Read the model definition and answer for the solid it produces. Units are mm, in the model's axes. Face numbers are marked on the shaded views. Give positions to 0.01 mm unless a question says otherwise; leave off trailing zeros. Order: outer loops, then holes, each group sorted by start corner. A loop starts at its lowest first (then second) coordinate and runs counter-clockwise, first axis right, second up. Notation, with made-up numbers: (-34.75, 55.25) - (-16.75, 55.25) arc R11 cw to (-16.75, 70.25) - close; hole circle Ø9 at (53, -31.75). An arc over 180 degrees is marked (long way). Return JSON: item names as keys, results as strings.
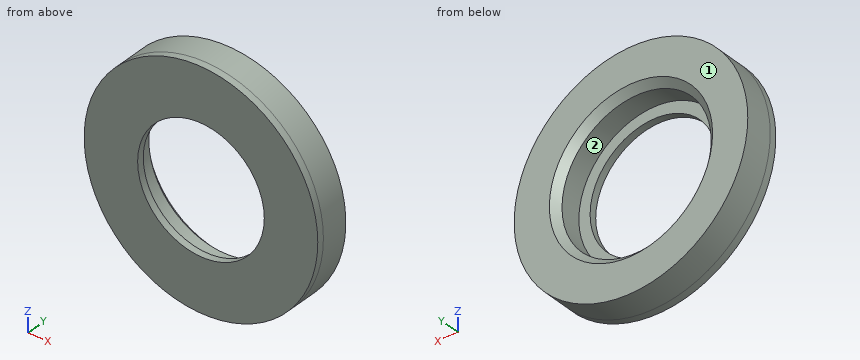
Autodesk Inventor part; units mm, degrees
ref_plane "YZ Plane" through (0, 0, 0) normal (1, 0, 0) x (0, 1, 0)
ref_plane "XZ Plane" through (0, 0, 0) normal (0, 1, 0) x (-1, 0, 0)
ref_plane "XY Plane" through (0, 0, 0) normal (0, 0, 1) x (1, 0, 0)
sketch "Sketch1" plane through (0, 0, 0) normal (0, 1, 0) x (-1, 0, 0)
  circle A0 centre (0, 0) radius 5.3
  circle A1 centre (0, 0) radius 8.3
  dimension "d0" = 10.6
  dimension "d1" = 3
extrude "Extrusion1" add sketch "Sketch1" along normal blind 2
sketch "Sketch2" plane through (0, 0, 0) normal (0, -1, 0) x (1, 0, 0)
  circle A0 centre (0, 0) radius 4.5
  circle A1 centre (0, 0) radius 8.3
  dimension "d4" = 9
extrude "Extrusion2" add sketch "Sketch2" along normal blind 0.5
chamfer "Chamfer1" distance 0.5 angle 45 1 edges at (5.3, 2, 0)
properties part number "623_flange"
Q1. A cutting plane is placed at D-D (x = -7). Write down the section's boundary in (y, z), and give its area (3 significant figures).
Values:
{"outline": "(-0.5, -4.46) - (2, -4.46) - (2, 4.46) - (-0.5, 4.46) - close", "area": "22.3 mm²"}
Q2. A cutting plane is placed at C-C (y = 0.3). Write down the section's boundary in (x, z), and give its area (3 significant figures).
Values:
{"outline": "circle Ø16.6 at (0, 0); hole circle Ø10.6 at (0, 0)", "area": "128 mm²"}
Q3. A cutting plane is placed at A-A (z = 0). Write down the section's boundary in (x, y).
Values:
{"outline": "(-8.3, -0.5) - (-4.5, -0.5) - (-4.5, 0) - (-5.3, 0) - (-5.3, 1.5) - (-5.8, 2) - (-8.3, 2) - close; (4.5, -0.5) - (8.3, -0.5) - (8.3, 2) - (5.8, 2) - (5.3, 1.5) - (5.3, 0) - (4.5, 0) - close"}
Q4. Given pin 1 (8.5 mm diameter, centred on x = 0, z = -1.5, fed in from +Y); pin 2 (1.5 mm diameter, centred on y = 1.5, z = -3, fed in from +X), each flat-ended and moving along its own axis, determine where each tip first touches the part or whether it passes through.
Values:
{"pin 1": "stops at y = 1.95", "pin 2": "stops at x = 7.99"}
Q5. A cutting plane is placed at B-B (x = 0). Write down the section's boundary in (y, z), and give its area (4 significant figures).
Values:
{"outline": "(-0.5, -8.3) - (2, -8.3) - (2, -5.8) - (1.5, -5.3) - (0, -5.3) - (0, -4.5) - (-0.5, -4.5) - close; (-0.5, 4.5) - (0, 4.5) - (0, 5.3) - (1.5, 5.3) - (2, 5.8) - (2, 8.3) - (-0.5, 8.3) - close", "area": "15.55 mm²"}
Q6. Consider L1, parallel to Z at x = 0, y = -0.4; L2, parallel to Z at x = 0, y = 1.1; L3, parallel to X at y = 1.05, z = 3.25. Determine where each line is inside the solid, lowest interval first.
Values:
{"L1": "z = -8.3 to -4.5, 4.5 to 8.3", "L2": "z = -8.3 to -5.3, 5.3 to 8.3", "L3": "x = -7.64 to -4.19, 4.19 to 7.64"}
Q7. Determine the mould class of the marked faces 1 and 2 for opening direction X: released by +X, released by -X, zero draft, split by the parting line, or undercut.
Values:
{"face 1": "zero draft", "face 2": "undercut"}
